Part print with two shaded views. Sizes in mm from the minimum x, y, z corner. A direction names the side the tool comes from. Round coordinates to 2 decimals unless told otherwise and drop trailing zeros. Loops run counter-clockwise (first coordinate to the right, second up) from the corner with the lowest first, then second, coordinate; pieces in that order, holes last. Notation, with made-up numbers: M 56.5,-26 L 69.5,-26 A16 cw 69.5,-10 Z; hole C 62,12.5 d2. An arc over 180 degrees is marked long. Put each result on its own line as item: value. Start each with the question number.
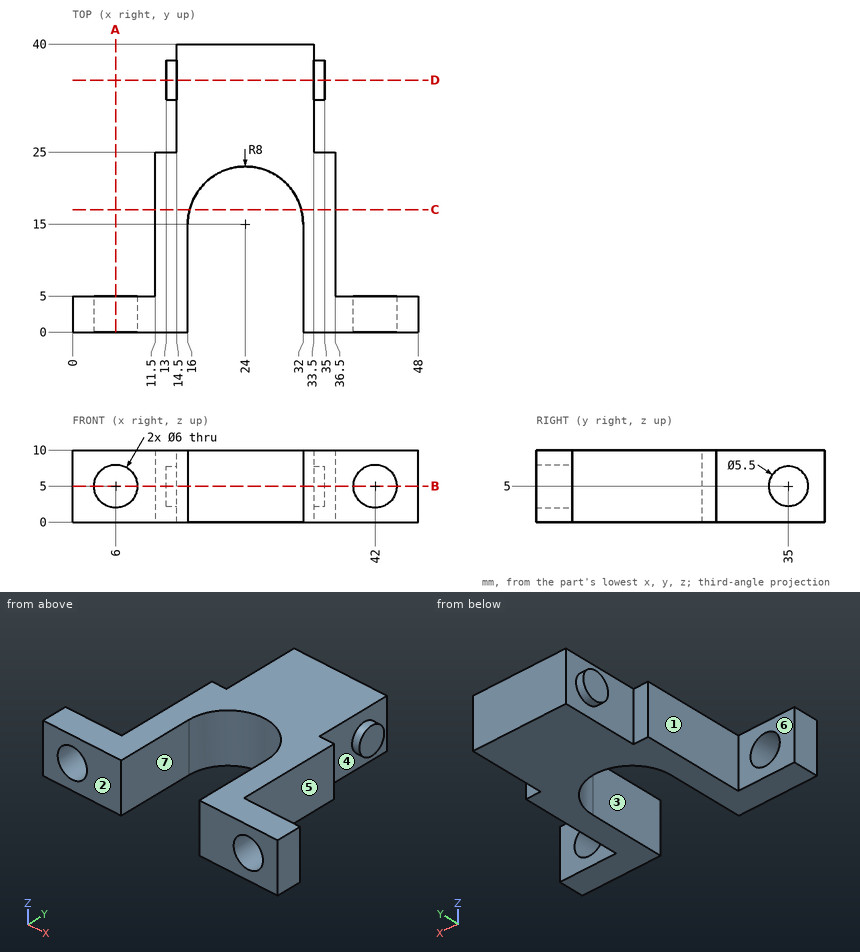
(1) Drill centre lines: line 1 along X through (y, z) = (2.9, 5); line 2 along Z through (x, y) = (6, 3.9); line 3 along X through (y, z) = (15, 9.5). Where is each one in solid material? Low to high.
(2) Tool access for the marked faces 4, 5, 6 and 7: list every direction of +Z, -Z, +X, -X, +Y, -Y with a clear straight run to the whole face (end or side of a thin tool).
(3) Cut at B-B on z = 5. Count the separate pieces of the cut face and the enclosed holes in it, and give its area (3 significant figures).
(4) Flat gauge pins, fed straight in: pin 1 Ø4.5 at (y, z) = (36, 4.5) entering from +X; pin 2 Ø3 at (x, z) = (11, 8) entering from +Y; pin 3 Ø3 at (y, z) = (33, 2.5) entering from -X. Where does each tip first touch, or does it go through?
(5) Mould opens along X. For the marked faces 1, 2 and 3 say: +X half, -X half, draft (parallel to the pull), parting line (faces both ways), or undercut.
(6) Cut at A-A on x = 6. List the corners of the cut face in (y, z).
(7) Cut at C-C on y = 17. List the corners of the cut face in (x, z), and give its area (3 significant figures).
(8) Cut at D-D on y = 35. List the corners of the cut face in (x, z), and give its area (4 significant figures).
Taken from the geometry:
1. line 1: 0 to 3, 9 to 16, 32 to 39, 45 to 48
1. line 2: 0 to 2, 8 to 10
1. line 3: 11.5 to 16, 32 to 36.5
2. face 4: +X
2. face 5: +Z, -Z, +X, +Y
2. face 6: +Z, -Z, -X, +Y
2. face 7: +Z, -Z, -Y
3. separate pieces: 3
3. enclosed holes: 0
3. area: 641 mm2
4. pin 1: x = 35
4. pin 2: y = 25
4. pin 3: x = 13
5. face 1: -X half
5. face 2: draft
5. face 3: undercut
6. outline: M 0,0 L 5,0 L 5,2 L 0,2 Z; M 0,8 L 5,8 L 5,10 L 0,10 Z
7. outline: M 11.5,0 L 16.25,0 L 16.25,10 L 11.5,10 Z; M 31.75,0 L 36.5,0 L 36.5,10 L 31.75,10 Z
7. area: 95.1 mm2
8. outline: M 13,2.25 L 14.5,2.25 L 14.5,0 L 33.5,0 L 33.5,2.25 L 35,2.25 L 35,7.75 L 33.5,7.75 L 33.5,10 L 14.5,10 L 14.5,7.75 L 13,7.75 Z
8. area: 206.5 mm2
